The listing builds one solid part. Answer for the finished solid, in the listing's coordinates (mm). A direction names the side the tool comes from. Coordinates: 2 decimals unless noted, no trailing zeros. Write each loop counter-clockwise with the first axis right and the second up, starting at its lowest first coordinate (ties: lowest second). Pieces come first, ordered by that corner, then holes.
from build123d import *

# Parameters (mm, degrees)
BOSS_EXTRUDE1_DEPTH = 1.27
BOSS_EXTRUDE2_DEPTH = 2.54
SKETCH2_W           = 17.018
SKETCH2_H           = 17.018
CUT_EXTRUDE1_DEPTH  = 1.778


with BuildPart() as part:
    # Sketch1 → Boss-Extrude1 (new body)
    with BuildSketch(Plane.XY):
        with BuildLine():
            Line((5.692726154, -53.086), (-12.087273846, -53.086))
            ThreePointArc((-12.087273846, -53.086), (-14.60174556, -52.044471714), (-15.643273846, -49.53))
            Line((-15.643273846, -49.53), (-15.643273846, -31.75))
            ThreePointArc((-15.643273846, -31.75), (-14.60174556, -29.235528286), (-12.087273846, -28.194))
            Line((-12.087273846, -28.194), (5.692726154, -28.194))
            ThreePointArc((5.692726154, -28.194), (8.207197868, -29.235528286), (9.248726154, -31.75))
            Line((9.248726154, -31.75), (9.248726154, -49.53))
            ThreePointArc((9.248726154, -49.53), (8.207197868, -52.044471714), (5.692726154, -53.086))
        make_face()
        with BuildLine():
            ThreePointArc((5.692726154, -50.419), (6.321344082, -50.158617928), (6.581726154, -49.53))
            Line((6.581726154, -49.53), (6.581726154, -31.75))
            ThreePointArc((6.581726154, -31.75), (6.321344082, -31.121382072), (5.692726154, -30.861))
            Line((5.692726154, -30.861), (-12.087273846, -30.861))
            ThreePointArc((-12.087273846, -30.861), (-12.715891775, -31.121382072), (-12.976273846, -31.75))
            Line((-12.976273846, -31.75), (-12.976273846, -49.53))
            ThreePointArc((-12.976273846, -49.53), (-12.715891775, -50.158617928), (-12.087273846, -50.419))
            Line((-12.087273846, -50.419), (5.692726154, -50.419))
        make_face(mode=Mode.SUBTRACT)
    extrude(amount=-BOSS_EXTRUDE1_DEPTH)

    # Sketch1_3 → Boss-Extrude2 (add)
    with BuildSketch(Plane.XY):
        with BuildLine():
            Line((5.692726154, -50.419), (-12.087273846, -50.419))
            ThreePointArc((-12.087273846, -50.419), (-12.715891775, -50.158617928), (-12.976273846, -49.53))
            Line((-12.976273846, -49.53), (-12.976273846, -31.75))
            ThreePointArc((-12.976273846, -31.75), (-12.715891775, -31.121382072), (-12.087273846, -30.861))
            Line((-12.087273846, -30.861), (5.692726154, -30.861))
            ThreePointArc((5.692726154, -30.861), (6.321344082, -31.121382072), (6.581726154, -31.75))
            Line((6.581726154, -31.75), (6.581726154, -49.53))
            ThreePointArc((6.581726154, -49.53), (6.321344082, -50.158617928), (5.692726154, -50.419))
        make_face()
    extrude(amount=-BOSS_EXTRUDE2_DEPTH)

    # Sketch2 → Cut-Extrude1 (cut)
    with BuildSketch(Plane(origin=(0, 0, -2.54), x_dir=(-1, 0, 0), z_dir=(0, 0, -1))):
        with Locations((3.197273846, -40.64)):
            Rectangle(SKETCH2_W, SKETCH2_H)
    extrude(amount=-CUT_EXTRUDE1_DEPTH, mode=Mode.SUBTRACT)


solid = part.part
Q1. The part is cut by section B-B, the plane y = -35. Write down the section's boundary in (x, z).
Answers below:
outline: (-15.64, -1.27) - (-12.98, -1.27) - (-12.98, -2.54) - (-11.71, -2.54) - (-11.71, -0.76) - (5.31, -0.76) - (5.31, -2.54) - (6.58, -2.54) - (6.58, -1.27) - (9.25, -1.27) - (9.25, 0) - (-15.64, 0) - close
Q2. The part is cut by section A-A, the plane z = -1.6. Write down the section's boundary in (x, y).
Answers below:
outline: (-12.98, -49.53) arc R0.89 ccw to (-12.09, -50.42) - (5.69, -50.42) arc R0.89 ccw to (6.58, -49.53) - (6.58, -31.75) arc R0.89 ccw to (5.69, -30.86) - (-12.09, -30.86) arc R0.89 ccw to (-12.98, -31.75) - close; hole (-11.71, -49.15) - (5.31, -49.15) - (5.31, -32.13) - (-11.71, -32.13) - close
Q3. The part is cut by section D-D, the plane x = 7. Write down the section's boundary in (y, z), then the cut area to 3 significant figures.
Answers below:
outline: (-52.84, -1.27) - (-28.44, -1.27) - (-28.44, 0) - (-52.84, 0) - close
area: 31.0 mm2
Q4. Which of the six approach directions +Z, -Z, +X, -X, +Y, -Y give full straight-line access (tool end or side, diameter ignored) to faces 1 (the face through (-3, -30.861, -2)), 2 (the face through (6.582, -41, -2)), 3 (the face through (-12.976, -41, -2)), 4 (the face through (-12.723, -31.128, -1.896))?
Answers below:
face 1: -Z, +X, -X, +Y
face 2: -Z, +X, +Y, -Y
face 3: -Z, -X, +Y, -Y
face 4: -Z, -X, +Y
Q5. The part is cut by section C-C, the plane x = -5. Write down the section's boundary in (y, z).
Answers below:
outline: (-53.09, -1.27) - (-50.42, -1.27) - (-50.42, -2.54) - (-49.15, -2.54) - (-49.15, -0.76) - (-32.13, -0.76) - (-32.13, -2.54) - (-30.86, -2.54) - (-30.86, -1.27) - (-28.19, -1.27) - (-28.19, 0) - (-53.09, 0) - close
Q6. Given pin 1 (12.5 mm diameter, centred on x = -4, y = -43.5, fed in from -Z); pin 2 (1 mm diameter, centred on x = -8, y = -45, fed in from -Z); pin 3 (1.4 mm diameter, centred on x = -7, z = -2, fed in from +Y); pin 4 (0.9 mm diameter, centred on y = -37, z = -2, fed in from -X), each flat-ended and moving along its own axis, determine where each tip first touches the part or whether it passes through.
Answers below:
pin 1: stops at z = -2.54
pin 2: stops at z = -0.76
pin 3: stops at y = -30.86
pin 4: stops at x = -12.98
Q7. Determine the mould class of faces 5 (the face through (-3, -50.419, -2)), 6 (the face through (-3, -41, -0.762)), 7 (the face through (6.3, -31.1, -1.9)), 8 (the face through (-11.706, -41, -2)) for opening direction X: released by +X, released by -X, zero draft, split by the parting line, or undercut.
Answers below:
face 5: zero draft
face 6: undercut
face 7: released by +X
face 8: undercut
Q8. Find the intervals of material crossed by probe 1 along Y at (x, z) = (-11.5, -2.1); probe 2 along X at (y, z) = (-45.5, -0.9); probe 3 along Y at (x, z) = (4.75, -1.2), in increasing order.
Answers below:
probe 1: y = -50.42 to -49.15, -32.13 to -30.86
probe 2: x = -15.64 to -11.71, 5.31 to 9.25
probe 3: y = -53.09 to -49.15, -32.13 to -28.19
